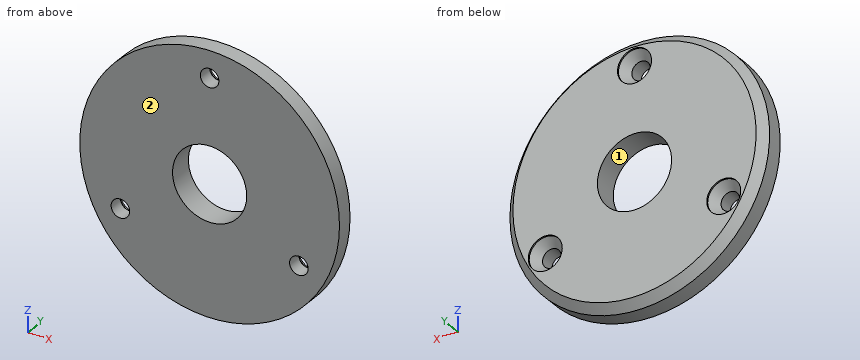
from build123d import *

# Parameters (mm, degrees)
CROQUIS1_R              = 31.5
CROQUIS1_R_2            = 9
SALIENTE_EXTRUIR1_DEPTH = 6
CHAFL_N1_SIZE           = 2
MATRIZC1_COUNT          = 3


with BuildPart() as part:
    # Croquis1 → Saliente-Extruir1 (new body)
    with BuildSketch(Plane(origin=(0, 0, 0), x_dir=(1, 0, 0), z_dir=(0, 1, 0))):
        Circle(CROQUIS1_R)
        Circle(CROQUIS1_R_2, mode=Mode.SUBTRACT)
    extrude(amount=SALIENTE_EXTRUIR1_DEPTH)

    # Chaflán1
    chafl_n1_edges = [part.edges().sort_by_distance(p)[0] for p in [
        (-31.5, 6, 0),
    ]]
    chamfer(chafl_n1_edges, length=CHAFL_N1_SIZE)

    # Croquis2 → Cortar-Revolución1 (revolve, cut)
    with BuildSketch(Plane(origin=(0, 0, 0), x_dir=(0, 0, -1), z_dir=(1, 0, 0))):
        Polygon((-25, 0), (-25, 6), (-20.875, 6), (-20.875, 5.64), (-22.75, 3.52), (-22.75, 0), align=None)
    cortar_revoluci_n1 = revolve(axis=Axis((0, 0, 25), (0, 1, 0)), mode=Mode.SUBTRACT)

    # MatrizC1: Cortar-Revolución1 ×3 about axis
    matrizc1_axis = Axis((0, 0, 0), (0, 1, 0))
    for i in range(1, MATRIZC1_COUNT):
        add(cortar_revoluci_n1.rotate(matrizc1_axis, i * 360 / MATRIZC1_COUNT), mode=Mode.SUBTRACT)


solid = part.part
Geometry check sheet. Reference: the model listing, model coordinates, mm. Face numbers are marked on the shaded views. Give positions to 0.01 mm unless a question says otherwise; leave off trailing zeros. Loops run counter-clockwise (first coordinate to the right, second up) from the corner with the lowest first, then second, coordinate; pieces in that order, holes last.
(1) Release check for a two-part mould opening along X. For the marked faces 1 and 2 record: released by +X, released by -X, zero draft, split by the parting line, or undercut.
From the geometry:
face 1: undercut
face 2: zero draft
(2) Section check A-A on x = 0. Record the cut outline in (y, z) (3 decimals).
From the geometry:
outline: (0, -31.5) - (4, -31.5) - (6, -29.5) - (6, -9) - (0, -9) - close; (0, 9) - (6, 9) - (6, 20.875) - (5.64, 20.875) - (3.52, 22.75) - (0, 22.75) - close; (0, 27.25) - (3.52, 27.25) - (5.64, 29.125) - (6, 29.125) - (6, 29.5) - (4, 31.5) - (0, 31.5) - close
(3) Depth check by flat-ended pin: pin 1 Ø7.5 at (x, z) = (0, 25) entering from +Y; pin 2 Ø9.5 at (x, z) = (21.65, -12.5) entering from -Y; pin 3 Ø1.5 at (x, y) = (13.5, 4.5) entering from +Z; pin 4 Ø2 at (y, z) = (3.5, -19) entering from +X. Enter the tip coordinate at first touch or a pass-through.
From the geometry:
pin 1: stops at y = 5.22
pin 2: stops at y = 0
pin 3: stops at z = 28.72
pin 4: stops at x = 25.85
(4) Section check D-D on z = -12.5. Count the separate pieces of the cut face and the enclosed holes in it, then the cut area to 3 significant figures.
From the geometry:
separate pieces: 3
enclosed holes: 0
area: 278 mm2
(5) Thickness scan on L1, parallel to Z at x = 0, y = 1.55; L2, parallel to X at y = 0.3, z = -12.5; L3, parallel to X at y = 5.95, z = -12.5. Record the ranges inside material, lowest first.
From the geometry:
L1: z = -31.5 to -9, 9 to 22.75, 27.25 to 31.5
L2: x = -28.91 to -23.9, -19.4 to 19.4, 23.9 to 28.91
L3: x = -26.78 to -25.78, -17.53 to 17.53, 25.78 to 26.78
(6) Section check C-C on y = 0.8. Record the cut outline in (x, z) (3 decimals).
From the geometry:
outline: circle Ø63 at (0, 0); hole circle Ø4.5 at (-21.651, -12.5); hole circle Ø18 at (0, 0); hole circle Ø4.5 at (0, 25); hole circle Ø4.5 at (21.651, -12.5)
(7) Section check B-B on z = 0. Record the cut outline in (x, y).
From the geometry:
outline: (-31.5, 0) - (-9, 0) - (-9, 6) - (-29.5, 6) - (-31.5, 4) - close; (9, 0) - (31.5, 0) - (31.5, 4) - (29.5, 6) - (9, 6) - close
